Verification items for the finished model (mm, model axes). A direction names the side the tool comes from. Coordinates: 2 decimals unless noted, no trailing zeros. Loops run counter-clockwise (first coordinate to the right, second up) from the corner with the lowest first, then second, coordinate; pieces in that order, holes last. Notation, with made-up numbers: M 29.25,54 L 66.25,54 A15 cw 66.25,79 Z; hole C 36.5,36.5 d3. An arc over 180 degrees is marked long. Write item = value, one per line. Start each with the question number.
```python
from build123d import *

# Parameters (mm, degrees)
SKETCH1_R           = 14.5
SKETCH1_R_2         = 1.5
SKETCH1_W           = 33
SKETCH1_H           = 21
BOSS_EXTRUDE1_DEPTH = 3
FILLET1_R           = 15
SKETCH2_R           = 1.5
CUT_EXTRUDE1_DEPTH  = 3
SKETCH4_R           = 1.75
CUT_EXTRUDE2_DEPTH  = 10


with BuildPart() as part:
    # Sketch1 → Boss-Extrude1 (new body)
    # profile 1 of 2: a face of its own
    with BuildSketch(Plane(origin=(0, 0, 0), x_dir=(1, 0, 0), z_dir=(0, 1, 0))):
        Circle(SKETCH1_R)
        with Locations(Location((-6.717514421, 6.717514421, 0), (0, 0, 270))):
            Circle(SKETCH1_R_2, mode=Mode.SUBTRACT)
        with Locations(Location((5.656854249, 5.656854249, 0), (0, 0, 270))):
            Circle(SKETCH1_R_2, mode=Mode.SUBTRACT)
        with Locations(Location((-5.656854249, -5.656854249, 0), (0, 0, 270))):
            Circle(SKETCH1_R_2, mode=Mode.SUBTRACT)
        with Locations(Location((6.717514421, -6.717514421, 0), (0, 0, 270))):
            Circle(SKETCH1_R_2, mode=Mode.SUBTRACT)
    # profile 2 of 2: a face of its own
    with BuildSketch(Plane(origin=(0, 0, 0), x_dir=(1, 0, 0), z_dir=(0, 1, 0))):
        with Locations((26.5, 0)):
            Rectangle(SKETCH1_W, SKETCH1_H)
    extrude(amount=BOSS_EXTRUDE1_DEPTH)

    # Fillet1
    fillet1_edges = [part.edges().sort_by_distance(p)[0] for p in [
        (10, 1.5, -10.5),
        (10, 1.5, 10.5),
    ]]
    fillet(fillet1_edges, radius=FILLET1_R)

    # Sketch2 → Cut-Extrude1 (cut)
    with BuildSketch(Plane(origin=(0, 3, 0), x_dir=(1, 0, 0), z_dir=(0, 1, 0))):
        with Locations(Location((23.75, 0, 0), (0, 0, 270))):
            Circle(SKETCH2_R)
        with Locations(Location((33.75, 0, 0), (0, 0, 270))):
            Circle(SKETCH2_R)
    extrude(amount=-CUT_EXTRUDE1_DEPTH, mode=Mode.SUBTRACT)

    # Sketch4 → Cut-Extrude2 (cut)
    with BuildSketch(Plane(origin=(0, 3, 0), x_dir=(1, 0, 0), z_dir=(0, 1, 0))):
        with Locations(Location((0, 0, 0), (0, 0, 270))):
            Circle(SKETCH4_R)
    extrude(amount=-CUT_EXTRUDE2_DEPTH, mode=Mode.SUBTRACT)


solid = part.part
```
Q1. Gauge pin test, flat end, axial feed: pin 1 (1.5 mm diameter, centred on x = 31, y = 1, fed in from +Z). Record the tip position at first contact, or that the pin passes through.
Q2. Scan lines: L1, parallel to X at y = 1.5, z = -0.75; L2, parallel to X at y = 1.5, z = 6.25; L3, parallel to X at y = 0.4, z = 7. Record each from-to range of solid material in increasing order. Write a range as [from, to].
Q3. Sectioned sample at D-D on y = 1.25. Record the cut outline in (x, z).
Q4. Mould release check, pull along X, two halves, no side actions. Record for faces 4 (the face through (14, 0, 0)), 5 (the face through (7.168, 1.479, 8.148)), 6 (the face through (43, 1, 0)): +X half, -X half, draft (parallel to the pull), parting line (faces both ways), or undercut.
Q5. Sectioned sample at C-C on x = 0. Record the cut outline in (y, z).
Q6. Sectioned sample at A-A on x = 33.75. Record the cut outline in (y, z), plus the area to 3 significant figures.
Q7. Sectioned sample at B-B on z = 0. Record the cut outline in (x, y), plus the area to 3 significant figures.
Q8. Set-up check for faces 1 (the face through (29, 1, -10.5)), 2 (the face through (-14.494, 1.479, -0.426)), 3 (the face through (29, 1, 10.5)): record each of +Z, -Z, +X, -X, +Y, -Y from which the full face is reachable in a straight line by a thin tool's end or side.
Solutions:
q1.pin_1 = 10.5
q2.L1 = [-14.48, -1.58], [1.58, 22.45], [25.05, 32.45], [35.05, 43]
q2.L2 = [-13.08, -7.03], [-4.28, 5.29], [8.14, 43]
q2.L3 = [-12.7, -6.32], [-4.99, 5.24], [8.19, 43]
q3.outline = M 7.29,-12.53 A15 cw 14.83,-10.5 L 43,-10.5 L 43,10.5 L 14.83,10.5 A15 cw 7.29,12.53 A14.5 ccw long Z; hole C -6.72,-6.72 d3; hole C -5.66,5.66 d3; hole C 0,0 d3.5; hole C 5.66,-5.66 d3; hole C 6.72,6.72 d3; hole C 23.75,0 d3; hole C 33.75,0 d3
q4.face_4 = draft
q4.face_5 = undercut
q4.face_6 = +X half
q5.outline = M 0,-14.5 L 3,-14.5 L 3,-1.75 L 0,-1.75 Z; M 0,1.75 L 3,1.75 L 3,14.5 L 0,14.5 Z
q6.outline = M 0,-10.5 L 3,-10.5 L 3,-1.5 L 0,-1.5 Z; M 0,1.5 L 3,1.5 L 3,10.5 L 0,10.5 Z
q6.area = 54.0 mm²
q7.outline = M -14.5,0 L -1.75,0 L -1.75,3 L -14.5,3 Z; M 1.75,0 L 22.25,0 L 22.25,3 L 1.75,3 Z; M 25.25,0 L 32.25,0 L 32.25,3 L 25.25,3 Z; M 35.25,0 L 43,0 L 43,3 L 35.25,3 Z
q7.area = 144 mm²
q8.face_1 = -Z, +X, +Y, -Y
q8.face_2 = +Y, -Y
q8.face_3 = +Z, +X, +Y, -Y
